```python
from build123d import *

# Parameters (mm, degrees)
BOSS_EXTRUDE1_DEPTH      = 60
BOSS_EXTRUDE1_DEPTH_BACK = 20


with BuildPart() as part:
    # Sketch1 → Boss-Extrude1 (new, two sides: drawn at the far end of the back side and taken through both)
    with BuildSketch(Plane(origin=(190.645148, 0, 0), x_dir=(0, 0, -1), z_dir=(1, 0, 0)).offset(-BOSS_EXTRUDE1_DEPTH_BACK)):
        with BuildLine():
            Line((-240.970904961, 189.163538159), (-246.970904961, 189.163538159))
            Line((-246.970904961, 189.163538159), (-246.970904961, 173.663538158))
            Line((-246.970904961, 173.663538158), (-240.970904961, 173.663538158))
            Line((-240.970904961, 173.663538158), (-240.970904961, 179.413538158))
            Line((-240.970904961, 179.413538158), (-241.970904961, 179.413538158))
            ThreePointArc((-241.970904961, 179.413538158), (-243.970904961, 181.413538158), (-241.970904961, 183.413538158))
            Line((-241.970904961, 183.413538158), (-240.970904961, 183.413538158))
            Line((-240.970904961, 183.413538158), (-240.970904961, 189.163538159))
        make_face()
    extrude(amount=BOSS_EXTRUDE1_DEPTH + BOSS_EXTRUDE1_DEPTH_BACK)


solid = part.part
```
Here's how the part is built. I have some questions about the finished solid (model axes, mm). Give positions to 0.01 mm unless a question says otherwise; leave off trailing zeros. Write each loop counter-clockwise with the first axis right and the second up, starting at its lowest first coordinate (ties: lowest second). Pieces come first, ordered by that corner, then holes.
(1) If I drill on L1, parallel to Y at x = 243, z = 242; L2, parallel to Y at x = 193, z = 243.15; L3, parallel to Z at x = 213, y = 181.25, over which ranges is the centre line in solid material (lowest first)?
Output values:
L1: y = 173.66 to 179.41, 183.41 to 189.16
L2: y = 173.66 to 179.8, 183.03 to 189.16
L3: z = 243.96 to 246.97
(2) Imagine slicing it at C-C, the plane y = 182.25. Write out the boundary of the cut face in (x, z).
Output values:
outline: (170.65, 243.79) - (250.65, 243.79) - (250.65, 246.97) - (170.65, 246.97) - close
(3) Thinking about a two-plate mould opening in Z: for faces 1 (the face through (170.645, 182, 245)), 2 (the face through (210, 176, 240.971)), 3 (the face through (210, 182, 246.971)), which applies, pulls with the +Z half, pulls with the -Z half, needs draft (parallel to the pull), parting line crosses it, or undercut?
Output values:
face 1: needs draft
face 2: pulls with the -Z half
face 3: pulls with the +Z half
(4) Imagine slicing it at B-B, the plane z = 242.7. Write out the boundary of the cut face in (x, y).
Output values:
outline: (170.65, 173.66) - (250.65, 173.66) - (250.65, 179.55) - (170.65, 179.55) - close; (170.65, 183.28) - (250.65, 183.28) - (250.65, 189.16) - (170.65, 189.16) - close
(5) Imagine slicing it at A-A, the plane x = 206. Write out the boundary of the cut face in (y, z), and give its area (3 significant figures).
Output values:
outline: (173.66, 240.97) - (179.41, 240.97) - (179.41, 241.97) arc R2 cw to (183.41, 241.97) - (183.41, 240.97) - (189.16, 240.97) - (189.16, 246.97) - (173.66, 246.97) - close
area: 82.7 mm2
